from build123d import *

# Parameters (mm, degrees)
F0_W      = 119.38
F0_H      = 60.96
F1_DEPTH  = 24.13
F3_DEPTH  = 90.932
F4_W      = 25.4
F4_H      = 10.16
F5_DEPTH  = 45.3898
F6_W      = 10.16
F6_H      = 35.56
F7_DEPTH  = 53.4162
F9_DEPTH  = 34.798
F11_DEPTH = 11.176
F12_R     = 6.35
F13_DEPTH = 58.166


with BuildPart() as f1:
    # F0 (on Top) → F1 (new body, symmetric)
    with BuildSketch(Plane.XY):
        Rectangle(F0_W, F0_H)
    extrude(amount=F1_DEPTH, both=True)

    # F2 (on face) → F3 (cut)
    with BuildSketch(Plane.YZ.offset(59.69)):
        Polygon((-30.48, -24.13), (-17.78, -24.13), (-17.78, 4.318), (17.78, 4.318), (17.78, -24.13), (30.48, -24.13), (30.48, 24.13), (-30.48, 24.13), align=None)
    extrude(amount=-F3_DEPTH, mode=Mode.SUBTRACT)

    # F4 (on face) → F5 (cut)
    with BuildSketch(Plane.YZ.offset(-31.242)):
        with Locations((0, 19.05)):
            Rectangle(F4_W, F4_H)
    extrude(amount=-F5_DEPTH, mode=Mode.SUBTRACT)

    # F6 (on face) → F7 (cut)
    with BuildSketch(Plane.XY.offset(24.13)):
        with Locations((-54.61, 0)):
            Rectangle(F6_W, F6_H)
    extrude(amount=-F7_DEPTH, mode=Mode.SUBTRACT)

    # F8 (on face) → F9 (cut)
    with BuildSketch(Plane.XY.offset(4.318)):
        Polygon((28.894137, 17.78), (59.69, 0), (59.69, 17.78), align=None)
        Polygon((59.69, -17.78), (59.69, 0), (28.894137, -17.78), align=None)
    extrude(amount=-F9_DEPTH, mode=Mode.SUBTRACT)

    # F10 (on face) → F11 (cut)
    with BuildSketch(Plane.XY.offset(4.318)):
        Polygon((40.386, 11.14517), (40.386, -11.14517), (59.69, 0), align=None)
    extrude(amount=-F11_DEPTH, mode=Mode.SUBTRACT)

    # F12 (on face) → F13 (cut)
    with BuildSketch(Plane.XZ.offset(17.78)):
        with Locations((3.81, -9.906)):
            Circle(F12_R)
    extrude(amount=-F13_DEPTH, mode=Mode.SUBTRACT)


solid = f1.part
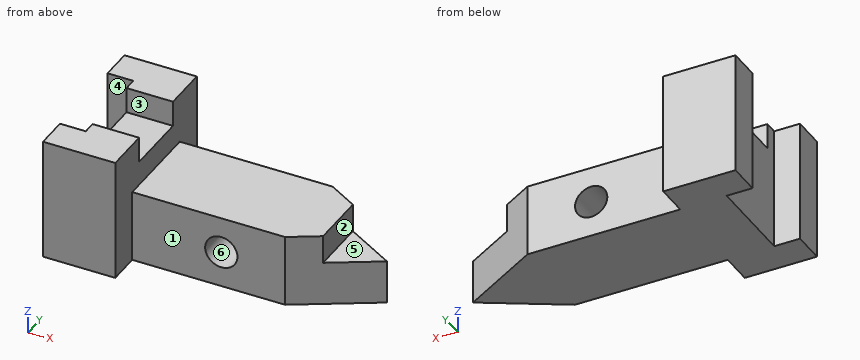
Geometry check sheet. Reference: the model listing, model coordinates, mm. Face numbers are marked on the shaded views. A direction names the side the tool comes from. Round coordinates to 2 decimals unless told otherwise and drop trailing zeros. Order: outer loops, then holes, each group sorted by start corner. A loop starts at its lowest first (then second) coordinate and runs counter-clockwise, first axis right, second up. Notation, with made-up numbers: M -22,-26.5 L -2,-26.5 A23 ccw -2,-1.5 Z; hole C 53.25,-14.75 d2. An arc over 180 degrees is marked long. Write each question's results on one line, items separated by ' | '. Start each with the question number.
1. Cross-section at B-B on z = 1.5. Record the boundary of the cut face in (x, y), plus the area to 3 significant figures.
2. Cross-section at C-C on x = -39. Record the boundary of the cut face in (y, z).
3. Cross-section at A-A on x = 3.81. Record the boundary of the cut face in (y, z).
4. Material ranges on L1, parallel to Z at x = 3.81, y = -10; L2, parallel to Y at x = 17, z = -21.5; L3, parallel to X at y = -24, z = -17, recorded low to high. Write a range as from..to.
5. Cross-section at D-D on z = -15. Record the boundary of the cut face in (x, y).
6. Set-up check for the marked faces 1, 2 and 3: record each of +Z, -Z, +X, -X, +Y, -Y from which the full face is reachable in a straight line by a thin tool's end or side.
7. Go/stop test with flat-tipped pins: P1, Ø14, axis at x = 14, z = -3, coming from the +Y side; P2, Ø11.5, axis at x = 3.81, z = -9.906, coming from the -Y side; P3, Ø3, axis at y = -14.5, z = 8, coming from the -X side; P4, Ø2, axis at x = 35, z = -5, coming from the -Y side. Record where each tip stops, or that it passes through.
8. Draft check along Z on the marked faces 4, 5 and 6. Enter one of: pulls with the +Z half, pulls with the -Z half, needs draft (parallel to the pull), parting line crosses it, or undercut.
Resolved:
1) outline: M -59.69,-30.48 L -31.24,-30.48 L -31.24,-17.78 L 28.89,-17.78 L 40.39,-11.15 L 40.39,11.15 L 28.89,17.78 L -31.24,17.78 L -31.24,30.48 L -59.69,30.48 L -59.69,17.78 L -49.53,17.78 L -49.53,-17.78 L -59.69,-17.78 Z | area: 3,840 mm2
2) outline: M -30.48,-24.13 L 30.48,-24.13 L 30.48,24.13 L 12.7,24.13 L 12.7,13.97 L -12.7,13.97 L -12.7,24.13 L -30.48,24.13 Z
3) outline: M -17.78,-24.13 L 17.78,-24.13 L 17.78,-16.26 L -17.78,-16.26 Z; M -17.78,-3.56 L 17.78,-3.56 L 17.78,4.32 L -17.78,4.32 Z
4) L1: -24.13..-16.26, -3.56..4.32 | L2: -17.78..17.78 | L3: -59.69..-31.24
5) outline: M -59.69,-30.48 L -31.24,-30.48 L -31.24,-17.78 L 0.02,-17.78 L 0.02,17.78 L -31.24,17.78 L -31.24,30.48 L -59.69,30.48 L -59.69,17.78 L -49.53,17.78 L -49.53,-17.78 L -59.69,-17.78 Z; M 7.6,-17.78 L 28.89,-17.78 L 59.69,0 L 28.89,17.78 L 7.6,17.78 Z
6) face 1: +Z, -Z, +X, -Y | face 2: +Z, +X, +Y, -Y | face 3: +Z, +X, -X
7) P1: y = 17.78 | P2: through | P3: x = -49.53 | P4: y = -14.83
8) face 4: needs draft | face 5: pulls with the +Z half | face 6: undercut
